Design review of the part built by this model. Coordinates are the model's own, in mm. A direction names the side the tool comes from. Round coordinates to 2 decimals unless told otherwise and drop trailing zeros. Write each loop counter-clockwise with the first axis right and the second up, starting at its lowest first coordinate (ties: lowest second). Pieces come first, ordered by that corner, then holes. Notation, with made-up numbers: (10, 68.5) -> (37, 68.5) arc R27 ccw to (37, 99.5) -> close; hole circle Ø1 at (-6.75, -36.75). An arc over 180 degrees is marked (long way). Write item = value, one per line. Start each with the question number.
Item 1: To check wall thickness, follow L1, parallel to X at y = -23, z = 1.6; L2, parallel to Y at x = -26.5, z = 1.85; L3, parallel to Y at x = -24, z = 2.35. State the ranges of each line that lie inside material, in increasing order.
Item 2: Add section B-B, the plane x = 17.5. State the section outline as (y, z) points, then the cut area to 3 significant figures.
Item 3: Mouldability with a two-part tool opening along Y and no side actions: class faces 4 (the flat face through (0, 0, 3)), 5 (the cylindrical face through (21.43, -33, 1.51)), 6 (the flat face through (23, -24.5, 1)) as released by +Y, released by -Y, zero draft, split by the parting line, or undercut.
Item 4: For pin 1 Ø1.5 at (x, z) = (20.5, 1.5) entering from -Y; pin 2 Ø1 at (x, z) = (16, 1) entering from -Y, all flat-tipped, find the tip position at first contact; note any pin that passes through.
Item 5: Machinability: for faces 1 (the cylindrical face through (33.5, 21.07, 1.51)), 2 (the cylindrical face through (-21.5, -33.07, 1.51)), 3 (the flat face through (25, -27, 1)), which of the approach directions +Z, -Z, +X, -X, +Y, -Y give a long, thin tool a straight path to every point of the face, cutting with its end or side? Answer none if there is none.
Item 6: Add section A-A, the plane y = -21. State the section outline as (x, z) points, then the cut area to 3 significant figures.
from build123d import *

# Parameters (mm, degrees)
F1_DEPTH = 3
F2_R     = 5
F3_R     = 1


with BuildPart() as f1:
    # F0 (on Top) → F1 (new body)
    with BuildSketch(Plane.XY):
        Polygon((35, -22.5), (35, 22.5), (-35, 22.5), (-35, -22.5), (-35, -34.5), (-20, -34.5), (-20, -24.5), (-25, -24.5), (-25, -29.5), (-30, -29.5), (-30, -9), (30, -9), (30, -29.5), (25, -29.5), (25, -24.5), (20, -24.5), (20, -34.5), (35, -34.5), align=None)
    extrude(amount=F1_DEPTH)

    # F2
    f2_edges = [f1.edges().sort_by_distance(p)[0] for p in [
        (-35, -34.5, 1.5),
        (-20, -34.5, 1.5),
        (-30, -9, 1.5),
        (35, -34.5, 1.5),
        (20, -34.5, 1.5),
        (35, 22.5, 1.5),
        (-35, 22.5, 1.5),
        (30, -9, 1.5),
    ]]
    fillet(f2_edges, radius=F2_R)

    # F3
    f3_edges = [f1.edges().sort_by_distance(p)[0] for p in [
        (0, 22.5, 3),
        (0, 22.5, 0),
        (0, -9, 3),
        (30, -21.75, 3),
        (0, -9, 0),
        (30, -21.75, 0),
    ]]
    fillet(f3_edges, radius=F3_R)


solid = f1.part
Result set:
q1.L1 = -35 to -30, 30 to 35
q1.L2 = -34.5 to -29.5, -9.23 to 22.5
q1.L3 = -34.33 to -24.5, -8.94 to 22.44
q2.outline = (-9, 1) arc R1 ccw to (-8, 0) -> (21.5, 0) arc R1 ccw to (22.5, 1) -> (22.5, 2) arc R1 ccw to (21.5, 3) -> (-8, 3) arc R1 ccw to (-9, 2) -> close
q2.area = 93.6 mm²
q3.face_4 = zero draft
q3.face_5 = released by -Y
q3.face_6 = undercut
q4.pin_1 = -32.81
q4.pin_2 = -9
q5.face_1 = +Z, -Z, +X, +Y
q5.face_2 = +Z, -Z, -Y
q5.face_3 = +Z, -Z
q6.outline = (-35, 1) arc R1 ccw to (-34, 0) -> (-31, 0) arc R1 ccw to (-30, 1) -> (-30, 2) arc R1 ccw to (-31, 3) -> (-34, 3) arc R1 ccw to (-35, 2) -> close; (30, 1) arc R1 ccw to (31, 0) -> (34, 0) arc R1 ccw to (35, 1) -> (35, 2) arc R1 ccw to (34, 3) -> (31, 3) arc R1 ccw to (30, 2) -> close
q6.area = 28.3 mm²
